Verification items for the finished model (mm, model axes). A direction names the side the tool comes from. Coordinates: 2 decimals unless noted, no trailing zeros. Loops run counter-clockwise (first coordinate to the right, second up) from the corner with the lowest first, then second, coordinate; pieces in that order, holes last. Notation, with made-up numbers: (-19, -3) -> (34, -3) arc R11 cw to (34, 16) -> close; hole circle Ø6 at (61.5, 12.5). An arc over 180 degrees is marked (long way). Answer as a JSON object with one key per item and string values. Group by question number.
Q1. Scan lines: L1, parallel to Z at x = -8.5, y = 6.5; L2, parallel to Z at x = 11.5, y = 0; L3, parallel to X at y = -7.5, z = -20.5. Record each from-to range of solid material in increasing order.
Q2. Set-up check for faces 4 (the flat face through (-1, -1, 36.451)), 5 (the flat face through (35.09, 0, -23)), 6 (the flat face through (-25, -9, -2.708)): record each of +Z, -Z, +X, -X, +Y, -Y from which the full face is reachable in a straight line by a thin tool's end or side.
Q3. Cross-section at D-D on y = 11. Record the boundary of the cut face in (x, z).
Q4. Cross-section at A-A on y = 0. Record the boundary of the cut face in (x, z), and give its area (3 significant figures).
Q5. Release check for a two-part mould opening along Z. For faces 1 (the flat face through (48.592, -1, -1)), 2 (the cylindrical face through (17.21, 0.46, -19.44)), 3 (the flat face through (-1, -1, -36.451)) record: released by +Z, released by -Z, zero draft, split by the parting line, or undercut.
Q6. Gauge pin test, flat ends, axial feed: pin 1 Ø8 at (y, z) = (-19.5, -21) entering from -X; pin 2 Ø2 at (y, z) = (1, -22) entering from -X. Record the tip position at first contact, or that the pin passes through.
Q7. Cross-section at B-B on x = -37. Record the boundary of the cut face in (y, z), and give its area (3 significant figures).
Q8. Cross-section at C-C on z = -11. Record the boundary of the cut face in (x, y), and give its area (3 significant figures).
```python
from build123d import *

# Parameters (mm, degrees)
F0_W     = 97.184672
F0_H     = 72.901874
F1_DEPTH = 44.5124
F3_DEPTH = 48.41849
F4_R     = 3.530572
F5_DEPTH = 35.26357


with BuildPart() as f1:
    # F0 (on Front) → F1 (new body, symmetric)
    with BuildSketch(Plane.XZ):
        Rectangle(F0_W, F0_H)
    extrude(amount=F1_DEPTH, both=True)

    # F2 (on face) → F3 (cut)
    with BuildSketch(Plane(origin=(-48.592336, 0, 0), x_dir=(0, -1, 0), z_dir=(-1, 0, 0))):
        with BuildLine():
            Line((44.5124, -2.707677), (-28.179571, -2.707677))
            ThreePointArc((-28.179571, -2.707677), (-41.152528, -15.680633), (-28.179571, -28.653589))
            Line((-28.179571, -28.653589), (44.5124, -28.653589))
            Line((44.5124, -28.653589), (44.5124, -2.707677))
        make_face()
    extrude(amount=-F3_DEPTH, mode=Mode.SUBTRACT)

    # F4 (on face) → F5 (cut)
    with BuildSketch(Plane(origin=(-0.173846, 0, 0), x_dir=(0, -1, 0), z_dir=(-1, 0, 0))):
        with Locations((0, -22.941379)):
            Circle(F4_R)
    extrude(amount=-F5_DEPTH, mode=Mode.SUBTRACT)


solid = f1.part
```
Computed values:
{
 "1": {"L1": "z = -36.45 to -28.65, -2.71 to 36.45", "L2": "z = -36.45 to -26.47, -19.41 to 36.45", "L3": "x = -0.17 to 48.59"},
 "2": {"face 4": "+Z, +X, -X, +Y, -Y", "face 5": "-X", "face 6": "-X, -Y"},
 "3": {"outline": "(-48.59, -36.45) -> (48.59, -36.45) -> (48.59, 36.45) -> (-48.59, 36.45) -> (-48.59, -2.71) -> (-0.17, -2.71) -> (-0.17, -28.65) -> (-48.59, -28.65) -> close"},
 "4": {"outline": "(-48.59, -36.45) -> (48.59, -36.45) -> (48.59, 36.45) -> (-48.59, 36.45) -> (-48.59, -2.71) -> (-0.17, -2.71) -> (-0.17, -19.41) -> (35.09, -19.41) -> (35.09, -26.47) -> (-0.17, -26.47) -> (-0.17, -28.65) -> (-48.59, -28.65) -> close", "area": "5,580 mm²"},
 "5": {"face 1": "zero draft", "face 2": "undercut", "face 3": "released by -Z"},
 "6": {"pin 1": "stops at x = -0.17", "pin 2": "stops at x = 35.09"},
 "7": {"outline": "(-44.51, -36.45) -> (44.51, -36.45) -> (44.51, 36.45) -> (-44.51, 36.45) -> (-44.51, -2.71) -> (28.18, -2.71) arc R12.97 cw to (28.18, -28.65) -> (-44.51, -28.65) -> close", "area": "4,340 mm²"},
 "8": {"outline": "(-48.59, 40.28) -> (-0.17, 40.28) -> (-0.17, -44.51) -> (48.59, -44.51) -> (48.59, 44.51) -> (-48.59, 44.51) -> close", "area": "4,550 mm²"}
}
